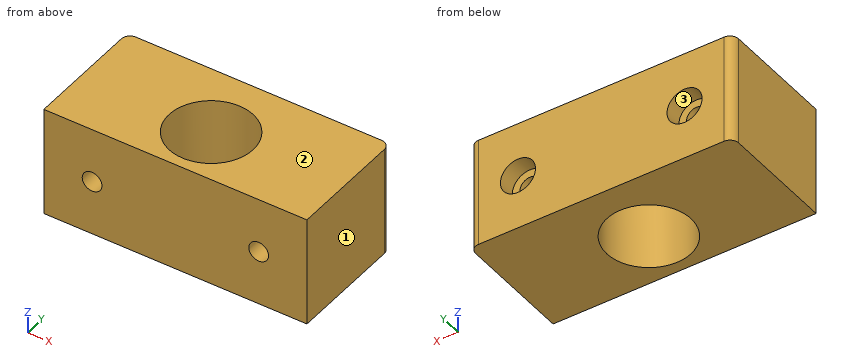
from build123d import *

# Parameters (mm, degrees)
SKETCH1_W                      = 60
SKETCH1_H                      = 25
BOSS_EXTRUDE1_DEPTH            = 28
SKETCH2_R                      = 9.5885
CUT_EXTRUDE1_DEPTH             = 26
CBORE_FOR_M4_SHCS1_D           = 4.5
CBORE_FOR_M4_SHCS1_CBORE_D     = 8
CBORE_FOR_M4_SHCS1_CBORE_DEPTH = 4
FILLET1_R                      = 2


with BuildPart() as part:
    # Sketch1 → Boss-Extrude1 (new body)
    with BuildSketch(Plane(origin=(0, 0, 0), x_dir=(1, 0, 0), z_dir=(0, 1, 0))):
        Rectangle(SKETCH1_W, SKETCH1_H)
    extrude(amount=BOSS_EXTRUDE1_DEPTH)

    # Sketch2 → Cut-Extrude1 (cut, through all)
    with BuildSketch(Plane.XY.offset(12.5)):
        with Locations((0, 12)):
            Circle(SKETCH2_R)
    extrude(amount=-CUT_EXTRUDE1_DEPTH, mode=Mode.SUBTRACT)

    # CBORE for M4 SHCS1 (through all)
    with Locations(Plane(origin=(0, 28, 0), x_dir=(1, 0, 0), z_dir=(0, 1, 0))):
        with Locations((-19, 0), (19, 0)):
            CounterBoreHole(CBORE_FOR_M4_SHCS1_D / 2, CBORE_FOR_M4_SHCS1_CBORE_D / 2, CBORE_FOR_M4_SHCS1_CBORE_DEPTH)

    # Fillet1
    fillet1_edges = [part.edges().sort_by_distance(p)[0] for p in [
        (-30, 28, 0),
        (30, 28, 0),
    ]]
    fillet(fillet1_edges, radius=FILLET1_R)


solid = part.part
Check sheet for the modelled part. Datum: model origin and axes. Units: mm. Face numbers are marked on the shaded views. Round coordinates to 2 decimals unless told otherwise and drop trailing zeros. Order: outer loops, then holes, each group sorted by start corner. A loop starts at its lowest first (then second) coordinate and runs counter-clockwise, first axis right, second up. Notation, with made-up numbers: M 20.25,22 L 35.25,22 A24 cw 35.25,57 Z; hole C -26.75,42 d5. An arc over 180 degrees is marked long. One line per item, written item: value. Start each with the question number.
1. Section check A-A on y = 12. Enter the section's corners in (x, z).
2. Gauge pin test, flat ends, axial feed: P1, Ø13, axis at x = 19, z = 0, coming from the -Y side; P2, Ø5, axis at x = 19, z = 0, coming from the +Y side. Record the tip position at first contact, or that the pin passes through.
3. Section check B-B on z = 0. Enter the section's corners in (x, y), and give its area (3 significant figures).
4. Section check C-C on x = 0. Enter the section's corners in (y, z), and give its area (3 significant figures).
5. Scan lines: line 1 along Z through (x, y) = (19, 13.5); line 2 along X through (y, z) = (20.75, -1); line 3 along Z through (x, y) = (-19, 25.7). Record each from-to range of solid material in increasing order.
6. Release check for a two-part mould opening along Z. For the marked faces 1, 2 and 3 record: released by +Z, released by -Z, zero draft, split by the parting line, or undercut.
7. Section check D-D on z = -6.5. Enter the section's corners in (x, y).
Results found:
1. outline: M -30,-12.5 L -9.59,-12.5 L -9.59,12.5 L -30,12.5 Z; M 9.59,-12.5 L 30,-12.5 L 30,12.5 L 9.59,12.5 Z; hole C -19,0 d4.5; hole C 19,0 d4.5
2. P1: y = 0
2. P2: y = 24
3. outline: M -30,0 L -21.25,0 L -21.25,24 L -23,24 L -23,28 L -28,28 A2 ccw -30,26 Z; M -16.75,0 L 16.75,0 L 16.75,24 L 15,24 L 15,28 L -15,28 L -15,24 L -16.75,24 Z; M 21.25,0 L 30,0 L 30,26 A2 ccw 28,28 L 23,28 L 23,24 L 21.25,24 Z; hole C 0,12 d19.18
3. area: 1,110 mm^2
4. outline: M 0,-12.5 L 2.41,-12.5 L 2.41,12.5 L 0,12.5 Z; M 21.59,-12.5 L 28,-12.5 L 28,12.5 L 21.59,12.5 Z
4. area: 221 mm^2
5. line 1: -12.5 to -2.25, 2.25 to 12.5
5. line 2: -30 to -21.02, -16.98 to -3.92, 3.92 to 16.98, 21.02 to 30
5. line 3: -12.5 to -4, 4 to 12.5
6. face 1: zero draft
6. face 2: released by +Z
6. face 3: undercut
7. outline: M -30,0 L 30,0 L 30,26 A2 ccw 28,28 L -28,28 A2 ccw -30,26 Z; hole C 0,12 d19.18
